Verification items for the finished model (mm, model axes). A direction names the side the tool comes from. Give positions to 0.01 mm unless a question says otherwise; leave off trailing zeros. Order: outer loops, then holes, each group sorted by start corner. A loop starts at its lowest first (then second) coordinate and runs counter-clockwise, first axis right, second up.
from build123d import *

# Parameters (mm, degrees)
SKETCH1_W             = 42.2
SKETCH1_H             = 42.2
SKETCH1_W_2           = 38.2
SKETCH1_H_2           = 38.2
SKETCH1_W_3           = 10
SKETCH1_H_3           = 10
BOSS_EXTRUDE1_DEPTH   = 2
M3X0_5_TAPPED_HOLE2_D = 2.5


with BuildPart() as part:
    # Sketch1 → Boss-Extrude1 (new body)
    # profile 1 of 5: a face of its own
    with BuildSketch(Plane(origin=(0, 0, 0), x_dir=(1, 0, 0), z_dir=(0, 1, 0))):
        with Locations((-63.025626343, 33.9108558)):
            Rectangle(SKETCH1_W, SKETCH1_H)
        with Locations((-63.025626343, 33.9108558)):
            Rectangle(SKETCH1_W_2, SKETCH1_H_2, mode=Mode.SUBTRACT)
    # profile 2 of 5: a face of its own
    with BuildSketch(Plane(origin=(0, 0, 0), x_dir=(1, 0, 0), z_dir=(0, 1, 0))):
        with Locations((-77.125626343, 48.0108558)):
            Rectangle(SKETCH1_W_3, SKETCH1_H_3)
    # profile 3 of 5: a face of its own
    with BuildSketch(Plane(origin=(0, 0, 0), x_dir=(1, 0, 0), z_dir=(0, 1, 0))):
        with Locations((-48.925626343, 48.0108558)):
            Rectangle(SKETCH1_W_3, SKETCH1_H_3)
    # profile 4 of 5: a face of its own
    with BuildSketch(Plane(origin=(0, 0, 0), x_dir=(1, 0, 0), z_dir=(0, 1, 0))):
        with Locations((-48.925626343, 19.8108558)):
            Rectangle(SKETCH1_W_3, SKETCH1_H_3)
    # profile 5 of 5: a face of its own
    with BuildSketch(Plane(origin=(0, 0, 0), x_dir=(1, 0, 0), z_dir=(0, 1, 0))):
        with Locations((-77.125626343, 19.8108558)):
            Rectangle(SKETCH1_W_3, SKETCH1_H_3)
    extrude(amount=BOSS_EXTRUDE1_DEPTH)

    # M3x0.5 Tapped Hole2 (through all)
    with Locations(Plane(origin=(0, 2, 0), x_dir=(1, 0, 0), z_dir=(0, 1, 0))):
        with Locations((-77.475626343, 48.3608558), (-48.575626343, 48.3608558), (-48.575626343, 19.4608558), (-77.475626343, 19.4608558)):
            Hole(M3X0_5_TAPPED_HOLE2_D / 2)


solid = part.part
(1) Section check C-C, the plane y = 1.35. Enter the section's corners in (x, z), then the cut area to 3 significant figures.
Solved:
outline: (-84.13, -55.01) - (-41.93, -55.01) - (-41.93, -12.81) - (-84.13, -12.81) - close; hole (-82.13, -43.01) - (-72.13, -43.01) - (-72.13, -53.01) - (-53.93, -53.01) - (-53.93, -43.01) - (-43.93, -43.01) - (-43.93, -24.81) - (-53.93, -24.81) - (-53.93, -14.81) - (-72.13, -14.81) - (-72.13, -24.81) - (-82.13, -24.81) - close; hole circle Ø2.5 at (-77.48, -48.36); hole circle Ø2.5 at (-77.48, -19.46); hole circle Ø2.5 at (-48.58, -48.36); hole circle Ø2.5 at (-48.58, -19.46)
area: 702 mm2
(2) Scan lines: line 1 (Z direction, x = -59.5, y = 0.3); line 2 (X direction, y = 0.45, z = -30.5); line 3 (Z direction, x = -52, y = 0.55). Record each from-to range of solid material in increasing order.
Solved:
line 1: z = -55.01 to -53.01, -14.81 to -12.81
line 2: x = -84.13 to -82.13, -43.93 to -41.93
line 3: z = -55.01 to -43.01, -24.81 to -12.81
(3) Release check for a two-part mould opening along X. For faces 1 (the flat face through (-53.926, 1, -20)), 2 (the flat face through (-72.126, 1, -48)), 3 (the flat face through (-63, 1, -12.811)), 4 (the flat face through (-84.126, 1, -34)) record: pulls with the +X half, pulls with the -X half, needs draft (parallel to the pull), parting line crosses it, or undercut.
Solved:
face 1: undercut
face 2: undercut
face 3: needs draft
face 4: pulls with the -X half
(4) Go/stop test with flat-tipped pins: pin 1 (3 mm diameter, centred on x = -69.5, z = -17, fed in from +Y); pin 2 (3 mm diameter, centred on x = -48.58, z = -19.46, fed in from -Y). Record where each tip stops, or that it passes through.
Solved:
pin 1: passes through
pin 2: stops at y = 0
(5) Set-up check for faces 5 (the flat face through (-77, 1, -24.811)), 6 (the flat face through (-53.7, 0, -43.4)): record each of +Z, -Z, +X, -X, +Y, -Y from which the full face is reachable in a straight line by a thin tool's end or side.
Solved:
face 5: +Y, -Y
face 6: +Z, -Z, +X, -X, -Y
(6) Section check B-B, the plane z = -45.5. Enter the section's corners in (x, y).
Solved:
outline: (-84.13, 0) - (-72.13, 0) - (-72.13, 2) - (-84.13, 2) - close; (-53.93, 0) - (-41.93, 0) - (-41.93, 2) - (-53.93, 2) - close
(7) Section check A-A, the plane x = -80. Enter the section's corners in (y, z), then the cut area to 3 significant figures.
Solved:
outline: (0, -55.01) - (2, -55.01) - (2, -43.01) - (0, -43.01) - close; (0, -24.81) - (2, -24.81) - (2, -12.81) - (0, -12.81) - close
area: 48.0 mm2
